from build123d import *

# Parameters (mm, degrees)
PAD006_DEPTH = 110
BOX051_W     = 117
BOX051_H     = 104
BOX051_DEPTH = 3
BOX050_W     = 118.2
BOX050_H     = 106.4
BOX050_DEPTH = 3


with BuildPart() as body004:
    # CopySketch011 → Pad006 (new body)
    with BuildSketch(Plane(origin=(0, 0, -162), x_dir=(1, 0, 0), z_dir=(0, -1, 0))):
        Polygon((0, 0), (2.01, 0), (19.87772, 170), (0, 170), align=None)
    extrude(amount=-PAD006_DEPTH)


with BuildPart() as cube043:
    # Box051 → Box051 (new body)
    with BuildSketch(Plane(origin=(0, 1.2, 0), x_dir=(1, 0, 0), z_dir=(0, 0, 1))):
        with Locations((58.5, 52)):
            Rectangle(BOX051_W, BOX051_H)
    extrude(amount=BOX051_DEPTH)


with BuildPart() as deckel_rahmen_cut:
    # Box050 → Box050 (new body)
    with BuildSketch(Plane.XY):
        with Locations((59.1, 53.2)):
            Rectangle(BOX050_W, BOX050_H)
    extrude(amount=BOX050_DEPTH)

    # Cut050: cut Cube043
    add(cube043.part, mode=Mode.SUBTRACT)


with BuildPart() as deckel_rahmen_cut_1:
    # Cut050 placement: moved
    add(deckel_rahmen_cut.part.moved(Location((0, 1.8, -19))))

    # Cut051: cut Body004
    add(body004.part, mode=Mode.SUBTRACT)


solid = deckel_rahmen_cut_1.part
The model under review builds one solid part; all positions refer to its coordinate system, in mm. A direction names the side the tool comes from. Give positions to 0.01 mm unless a question says otherwise; leave off trailing zeros. Order: outer loops, then holes, each group sorted by start corner. A loop starts at its lowest first (then second) coordinate and runs counter-clockwise, first axis right, second up. Notation, with made-up numbers: (0, 17.5) -> (31, 17.5) arc R13 cw to (31, 34.5) -> close; hole circle Ø10 at (44.25, 40). An arc over 180 degrees is marked (long way). Write item = value, one per line. Start each with the question number.
(1) For L1, parallel to Y at x = 42.5, z = -17.6; L2, parallel to X at y = 37.5, z = -17.2, list the stretches that pass through material, from the lowest coordinate up. Write a range as from..to.
(2) Draft analysis for pull direction Y (two halves, no side actions). For faces 1 (the flat face through (66, 3, -18)), 2 (the flat face through (66, 107, -18)), 3 (the flat face through (118.2, 54, -18)), 4 (the flat face through (67, 108.2, -18)), state which applies: +Y half, -Y half, draft (parallel to the pull), parting line (faces both ways), or undercut.
(3) Tool access review of faces 5 (the flat face through (117, 54, -18)), 6 (the flat face through (67, 1.8, -18)): name each direction out of +Z, -Z, +X, -X, +Y, -Y from which nothing blocks a thin tool from reaching the whole face with its end or side.
(4) Take a section at A-A (x = 29). Write out the cut boundary in (y, z).
(5) Take a section at C-C (y = 26). Write out the cut boundary in (x, z), plus the area to 3 significant figures.
(6) Take a section at B-B (z = -17.7). Write out the cut boundary in (x, y).
(7) For pin 1 Ø0.9 at (y, z) = (62.5, -18) entering from -X, flat-tipped, find the tip position at first contact; note if it passes through.
Returned:
q1.L1 = 1.8..3, 107..108.2
q1.L2 = 117..118.2
q2.face_1 = undercut
q2.face_2 = undercut
q2.face_3 = draft
q2.face_4 = +Y half
q3.face_5 = +Z, -Z, -X
q3.face_6 = +Z, -Z, +X, -X, -Y
q4.outline = (1.8, -19) -> (3, -19) -> (3, -16) -> (1.8, -16) -> close; (107, -19) -> (108.2, -19) -> (108.2, -16) -> (107, -16) -> close
q5.outline = (117, -19) -> (118.2, -19) -> (118.2, -16) -> (117, -16) -> close
q5.area = 3.60 mm²
q6.outline = (17.18, 1.8) -> (118.2, 1.8) -> (118.2, 108.2) -> (17.18, 108.2) -> (17.18, 107) -> (117, 107) -> (117, 3) -> (17.18, 3) -> close
q7.pin_1 = 117
